Read the model definition and answer for the solid it produces. Units are mm, in the model's axes. Face numbers are marked on the shaded views. A direction names the side the tool comes from. Give positions to 0.01 mm unless a question says otherwise; leave off trailing zeros. Order: outer loops, then holes, each group sorted by start corner. A loop starts at its lowest first (then second) coordinate and runs counter-clockwise, first axis right, second up. Notation, with made-up numbers: (3, 55) -> (16, 55) arc R16 ccw to (16, 74) -> close; hole circle Ø7 at (-16, 71). An arc over 180 degrees is marked (long way). One line per item, written item: value. Start each with the question number.
from build123d import *

# Parameters (mm, degrees)
SKETCH1_W           = 78
SKETCH1_H           = 93
BOSS_EXTRUDE1_DEPTH = 1.75
SKETCH2_R           = 1.8
CUT_EXTRUDE1_DEPTH  = 1.75
SKETCH3_W           = 58.25
SKETCH3_H           = 65.6
BOSS_EXTRUDE2_DEPTH = 16
FILLET1_R           = 1
SKETCH4_W           = 10.6
SKETCH4_H           = 7
BOSS_EXTRUDE3_DEPTH = 9.45
BOSS_EXTRUDE4_START = 2.25
BOSS_EXTRUDE4_DEPTH = 2.25
SKETCH6_W           = 11.2
SKETCH6_H           = 7.75
BOSS_EXTRUDE5_DEPTH = 2.25
SKETCH7_W           = 51.25
SKETCH7_H           = 58.6
CUT_EXTRUDE2_DEPTH  = 13.75
SKETCH8_R           = 2.5
BOSS_EXTRUDE6_DEPTH = 4.15
FILLET2_R           = 1


with BuildPart() as part:
    # Sketch1 → Boss-Extrude1 (new body)
    with BuildSketch(Plane(origin=(0, 0, 0), x_dir=(1, 0, 0), z_dir=(0, 1, 0))):
        Rectangle(SKETCH1_W, SKETCH1_H)
    extrude(amount=BOSS_EXTRUDE1_DEPTH)

    # Sketch2 → Cut-Extrude1 (cut)
    with BuildSketch(Plane(origin=(0, 1.75, 0), x_dir=(1, 0, 0), z_dir=(0, 1, 0))):
        with Locations(Location((-33.8, 38.6, 0), (0, 0, 270))):
            Circle(SKETCH2_R)
        with Locations(Location((33.8, 38.6, 0), (0, 0, 270))):
            Circle(SKETCH2_R)
        with Locations(Location((33.8, -38.6, 0), (0, 0, 270))):
            Circle(SKETCH2_R)
        with Locations(Location((-33.8, -38.6, 0), (0, 0, 270))):
            Circle(SKETCH2_R)
        with BuildLine():
            Line((-39, 36.5), (-39, 46.5))
            Line((-39, 46.5), (-29, 46.5))
            ThreePointArc((-29, 46.5), (-36.071067812, 43.571067812), (-39, 36.5))
        make_face()
        with BuildLine():
            Line((39, 36.5), (39, 46.5))
            Line((39, 46.5), (29, 46.5))
            ThreePointArc((29, 46.5), (36.071067812, 43.571067812), (39, 36.5))
        make_face()
        with BuildLine():
            Line((39, -36.5), (39, -46.5))
            Line((39, -46.5), (29, -46.5))
            ThreePointArc((29, -46.5), (36.071067812, -43.571067812), (39, -36.5))
        make_face()
        with BuildLine():
            Line((-39, -36.5), (-39, -46.5))
            Line((-39, -46.5), (-29, -46.5))
            ThreePointArc((-29, -46.5), (-36.071067812, -43.571067812), (-39, -36.5))
        make_face()
    extrude(amount=-CUT_EXTRUDE1_DEPTH, mode=Mode.SUBTRACT)

    # Sketch3 → Boss-Extrude2 (add)
    with BuildSketch(Plane(origin=(0, 1.75, 0), x_dir=(1, 0, 0), z_dir=(0, 1, 0))):
        with Locations((0, 3.7)):
            Rectangle(SKETCH3_W, SKETCH3_H)
    extrude(amount=BOSS_EXTRUDE2_DEPTH)

    # Fillet1
    fillet1_edges = [part.edges().sort_by_distance(p)[0] for p in [
        (0, 17.75, -36.5),
        (29.125, 9.75, -36.5),
        (29.125, 17.75, -3.7),
        (29.125, 9.75, 29.1),
        (0, 17.75, 29.1),
        (-29.125, 9.75, 29.1),
        (-29.125, 17.75, -3.7),
        (-29.125, 9.75, -36.5),
    ]]
    fillet(fillet1_edges, radius=FILLET1_R)

    # Sketch4 → Boss-Extrude3 (add)
    with BuildSketch(Plane(origin=(0, 1.75, 0), x_dir=(1, 0, 0), z_dir=(0, 1, 0))):
        with Locations((-19.825, -35.45)):
            Rectangle(SKETCH4_W, SKETCH4_H)
    extrude(amount=BOSS_EXTRUDE3_DEPTH)

    # Sketch5 → Boss-Extrude4 (add)
    with BuildSketch(Plane(origin=(0, 1.75, 0), x_dir=(1, 0, 0), z_dir=(0, 1, 0)).offset(BOSS_EXTRUDE4_START)):
        with BuildLine():
            Line((-28.125, -30.6), (28.125, -30.6))
            ThreePointArc((28.125, -30.6), (29.892766953, -29.867766953), (30.625, -28.1))
            Line((30.625, -28.1), (30.625, 35.5))
            ThreePointArc((30.625, 35.5), (29.892766953, 37.267766953), (28.125, 38))
            Line((28.125, 38), (-28.125, 38))
            ThreePointArc((-28.125, 38), (-29.892766953, 37.267766953), (-30.625, 35.5))
            Line((-30.625, 35.5), (-30.625, -28.1))
            ThreePointArc((-30.625, -28.1), (-29.892766953, -29.867766953), (-28.125, -30.6))
        make_face()
        with BuildLine():
            ThreePointArc((-29.125, 35.5), (-28.832106781, 36.207106781), (-28.125, 36.5))
            Line((-28.125, 36.5), (28.125, 36.5))
            ThreePointArc((28.125, 36.5), (28.832106781, 36.207106781), (29.125, 35.5))
            Line((29.125, 35.5), (29.125, -28.1))
            ThreePointArc((29.125, -28.1), (28.832106781, -28.807106781), (28.125, -29.1))
            Line((28.125, -29.1), (-28.125, -29.1))
            ThreePointArc((-28.125, -29.1), (-28.832106781, -28.807106781), (-29.125, -28.1))
            Line((-29.125, -28.1), (-29.125, 35.5))
        make_face(mode=Mode.SUBTRACT)
    extrude(amount=-BOSS_EXTRUDE4_DEPTH)

    # Sketch6 → Boss-Extrude5 (add)
    with BuildSketch(Plane(origin=(0, 1.75, 0), x_dir=(1, 0, 0), z_dir=(0, 1, 0))):
        with Locations((19.275, -34.475)):
            Rectangle(SKETCH6_W, SKETCH6_H)
    extrude(amount=BOSS_EXTRUDE5_DEPTH)

    # Sketch7 → Cut-Extrude2 (cut)
    with BuildSketch(Plane.XZ):
        with Locations((0, -3.7)):
            Rectangle(SKETCH7_W, SKETCH7_H)
    extrude(amount=-CUT_EXTRUDE2_DEPTH, mode=Mode.SUBTRACT)

    # Sketch8 → Boss-Extrude6 (add)
    with BuildSketch(Plane(origin=(0, 4, 0), x_dir=(1, 0, 0), z_dir=(0, 1, 0))):
        with Locations(Location((19.222552854, -33.536468805, 0), (0, 0, 90))):
            Circle(SKETCH8_R)
    extrude(amount=BOSS_EXTRUDE6_DEPTH)

    # Fillet2
    fillet2_edges = [part.edges().sort_by_distance(p)[0] for p in [
        (19.222552854, 8.15, 36.036468805),
    ]]
    fillet(fillet2_edges, radius=FILLET2_R)


solid = part.part
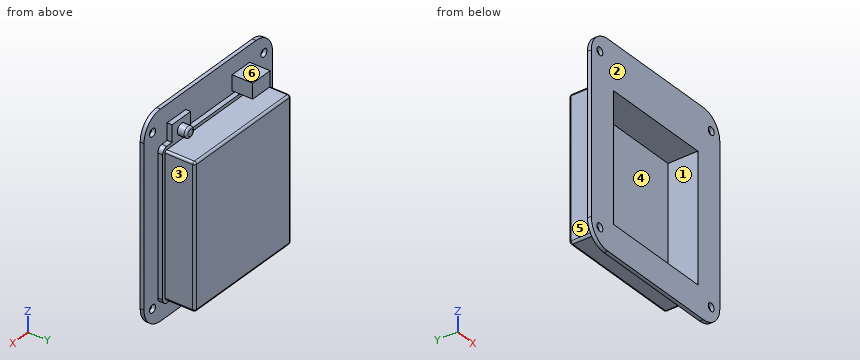
Item 1: Find section A-A on y = 2.75. Write down the section's boundary in (x, z) (3 decimals).
Item 2: Find the intervals of material crossed by line 1 (X direction, y = 5.5, z = 18.5) (3 decimals); line 2 (X direction, y = 3.75, z = -20) (3 decimals); line 3 (X direction, y = 0.45, z = 38.6), in increasing order. Write a range as from..to.
Item 3: Flat-ended cylindrical pins translate along their axes: pin 1 (1.1 mm diameter, centred on y = 2.5, z = 35.5, fed in from +X) (3 decimals); pin 2 (7 mm diameter, centred on x = -11.5, y = 4, fed in from -Z); pin 3 (1.5 mm diameter, centred on y = 11.5, z = 26, fed in from -X) (3 decimals); pin 4 (4.5 mm diameter, centred on x = 33.8, z = -38.6, fed in from +Y). Find the tip coordinate at first contact, or state that the pin passes through.
Item 4: A tool of negligible diameter and unlimited length cuts with its end or side. For the marked faces 1, 2 and 3, from which of +Z, -Z, +X, -X, +Y, -Y can it reach the whole face along a straight path? Write none if from no direction.
Item 5: Find section B-B on x = 33.8. Write down the section's boundary in (y, z), then the cut area to 3 significant figures.
Item 6: For a pull along Z with two mould halves and no side action, classify the marked faces 4, 5 and 6 as +Z half, -Z half, draft (parallel to the pull), parting line (faces both ways), or undercut.
Item 7: Find section C-C on z = 18. Write down the section's boundary in (x, y) (3 decimals).
Item 8: Find section D-D on x = 9. Write down the section's boundary in (y, z).
Checks:
1. outline: (-30.625, -35.5) arc R2.5 ccw to (-28.125, -38) -> (28.125, -38) arc R2.5 ccw to (30.625, -35.5) -> (30.625, 28.1) arc R2.5 ccw to (28.125, 30.6) -> (24.875, 30.6) -> (24.875, 38.35) -> (13.675, 38.35) -> (13.675, 30.6) -> (-28.125, 30.6) arc R2.5 ccw to (-30.625, 28.1) -> close; (-25.125, 31.95) -> (-14.525, 31.95) -> (-14.525, 38.95) -> (-25.125, 38.95) -> close; hole (-25.625, -33) -> (25.625, -33) -> (25.625, 25.6) -> (-25.625, 25.6) -> close
2. line 1: -29.125..-25.625, 25.625..29.125
2. line 2: -30.625..-25.625, 25.625..30.625
2. line 3: -38.78..-35.6, -32..32, 35.6..38.78
3. pin 1: x = 24.875
3. pin 2: z = -46.5
3. pin 3: x = -29.125
3. pin 4: y = 1.75
4. face 1: -Y
4. face 2: +Z, -Z, +X, -X, -Y
4. face 3: +Z, -Z, +X, +Y
5. outline: (0, -45.27) -> (1.75, -45.27) -> (1.75, -40.4) -> (0, -40.4) -> close; (0, -36.8) -> (1.75, -36.8) -> (1.75, 36.8) -> (0, 36.8) -> close; (0, 40.4) -> (1.75, 40.4) -> (1.75, 45.27) -> (0, 45.27) -> close
5. area: 146 mm2
6. face 4: undercut
6. face 5: draft
6. face 6: +Z half
7. outline: (-39, 0) -> (-25.625, 0) -> (-25.625, 13.75) -> (25.625, 13.75) -> (25.625, 0) -> (39, 0) -> (39, 1.75) -> (30.625, 1.75) -> (30.625, 4) -> (29.125, 4) -> (29.125, 16.75) arc R1 ccw to (28.125, 17.75) -> (-28.125, 17.75) arc R1 ccw to (-29.125, 16.75) -> (-29.125, 4) -> (-30.625, 4) -> (-30.625, 1.75) -> (-39, 1.75) -> close
8. outline: (0, -46.5) -> (1.75, -46.5) -> (1.75, -38) -> (4, -38) -> (4, -36.5) -> (16.75, -36.5) arc R1 ccw to (17.75, -35.5) -> (17.75, 28.1) arc R1 ccw to (16.75, 29.1) -> (4, 29.1) -> (4, 30.6) -> (1.75, 30.6) -> (1.75, 46.5) -> (0, 46.5) -> (0, 25.6) -> (13.75, 25.6) -> (13.75, -33) -> (0, -33) -> close
